Design review of the part built by this model. Coordinates are the model's own, in mm. A direction names the side the tool comes from. Coordinates: 2 decimals unless noted, no trailing zeros. Write each loop counter-clockwise with the first axis right and the second up, starting at its lowest first coordinate (ties: lowest second). Pieces come first, ordered by that corner, then holes. Notation, with made-up numbers: (40, 30) -> (67, 30) arc R30 cw to (67, 67) -> close; hole circle Ø11 at (-26.5, 9). An arc over 180 degrees is marked (long way). Answer in a Markdown table with one row per item. Add a question column.
Item 1: Take a section at C-C, the plane z = 2. Write out the cut boundary in (x, y) (3 decimals), and give its area (3 significant figures).
Item 2: For faces 1 (the face through (-6, -37, 0)), 2 (the face through (0.07, -28.574, 1.61)), list the 3-axis set-ups (+Z, -Z, +X, -X, +Y, -Y) from which the entire face can be reached by the end or side of a thin tool; tool diameter is ignored.
Item 3: Take a section at A-A, the plane x = 0. Write out the cut boundary in (y, z) (3 decimals), and give its area (3 significant figures).
Item 4: Draft analysis for pull direction Y (two halves, no side actions). For faces 3 (the face through (-12.7, -39, 2)), 4 (the face through (-0.07, -34.926, 1.61)), 5 (the face through (0.07, -73.024, 1.61)), 6 (the face through (0, 12.7, 2)), state which applies: released by +Y, released by -Y, zero draft, split by the parting line, or undercut.
Item 5: Take a section at B-B, the plane y = -55.5. Write out the cut boundary in (x, z) (3 decimals).
Item 6: To check wall thickness, follow line 1 (Y direction, x = 0, z = 0.75) (3 decimals); line 2 (X direction, y = -8, z = 0.9) (3 decimals); line 3 (Y direction, x = -2, z = 0.6). State the ranges of each line that lie inside material, in increasing order.
from build123d import *

# Parameters (mm, degrees)
SKETCH1_W           = 25.4
SKETCH1_H           = 101.6
SKETCH1_R           = 2.38125
BOSS_EXTRUDE1_DEPTH = 3.175
CUT_EXTRUDE1_DEPTH  = 4.175


with BuildPart() as part:
    # Sketch1 → Boss-Extrude1 (new body)
    with BuildSketch(Plane.XY):
        with Locations((0, -38.1)):
            Rectangle(SKETCH1_W, SKETCH1_H)
        with Locations((0, 6.35)):
            Circle(SKETCH1_R, mode=Mode.SUBTRACT)
        with Locations((0, -69.85)):
            Circle(SKETCH1_R, mode=Mode.SUBTRACT)
    extrude(amount=BOSS_EXTRUDE1_DEPTH)

    # Sketch2 → Cut-Extrude1 (cut, through all)
    with BuildSketch(Plane.XY.offset(3.175)):
        with BuildLine():
            Line((-3.175, -25.4), (-3.175, 6.35))
            ThreePointArc((-3.175, 6.35), (0, 9.525), (3.175, 6.35))
            Line((3.175, 6.35), (3.175, -25.4))
            ThreePointArc((3.175, -25.4), (0, -28.575), (-3.175, -25.4))
        make_face()
        with BuildLine():
            Line((-3.175, -69.85), (-3.175, -38.1))
            ThreePointArc((-3.175, -38.1), (0, -34.925), (3.175, -38.1))
            Line((3.175, -38.1), (3.175, -69.85))
            ThreePointArc((3.175, -69.85), (0, -73.025), (-3.175, -69.85))
        make_face()
    extrude(amount=-CUT_EXTRUDE1_DEPTH, mode=Mode.SUBTRACT)


solid = part.part
Answers:
| question | item | result |
|---|---|---|
| 1 | outline | (-12.7, -88.9) -> (12.7, -88.9) -> (12.7, 12.7) -> (-12.7, 12.7) -> close; hole (-3.175, -69.85) arc R3.175 ccw to (3.175, -69.85) -> (3.175, -38.1) arc R3.175 ccw to (-3.175, -38.1) -> close; hole (-3.175, -25.4) arc R3.175 ccw to (3.175, -25.4) -> (3.175, 6.35) arc R3.175 ccw to (-3.175, 6.35) -> close |
| 1 | area | 2,110 mm^2 |
| 2 | face 1 | -Z, +X, -X, +Y, -Y |
| 2 | face 2 | +Z, -Z |
| 3 | outline | (-88.9, 0) -> (-73.025, 0) -> (-73.025, 3.175) -> (-88.9, 3.175) -> close; (-34.925, 0) -> (-28.575, 0) -> (-28.575, 3.175) -> (-34.925, 3.175) -> close; (9.525, 0) -> (12.7, 0) -> (12.7, 3.175) -> (9.525, 3.175) -> close |
| 3 | area | 80.6 mm^2 |
| 4 | face 3 | zero draft |
| 4 | face 4 | undercut |
| 4 | face 5 | undercut |
| 4 | face 6 | released by +Y |
| 5 | outline | (-12.7, 0) -> (-3.175, 0) -> (-3.175, 3.175) -> (-12.7, 3.175) -> close; (3.175, 0) -> (12.7, 0) -> (12.7, 3.175) -> (3.175, 3.175) -> close |
| 6 | line 1 | y = -88.9 to -73.025, -34.925 to -28.575, 9.525 to 12.7 |
| 6 | line 2 | x = -12.7 to -3.175, 3.175 to 12.7 |
| 6 | line 3 | y = -88.9 to -72.32, -35.63 to -27.87, 8.82 to 12.7 |
